The listing builds one solid part. Answer for the finished solid, in the listing's coordinates (mm). Give positions to 0.01 mm unless a question says otherwise; leave off trailing zeros. Write each loop counter-clockwise with the first axis right and the second up, starting at its lowest first coordinate (ties: lowest second). Pieces come first, ordered by that corner, then holes.
```python
from build123d import *

# Parameters (mm, degrees)
SKETCH1_R           = 1.5
BOSS_EXTRUDE1_DEPTH = 2
FILLET1_R           = 8


with BuildPart() as part:
    # Sketch1 → Boss-Extrude1 (new body)
    with BuildSketch(Plane.XY):
        with BuildLine():
            Line((85, 40), (85, -45))
            Line((85, -45), (58.094750193, -45))
            ThreePointArc((58.094750193, -45), (0, -30), (-58.094750193, -45))
            Line((-58.094750193, -45), (-85, -45))
            Line((-85, -45), (-85, 40))
            ThreePointArc((-85, 40), (-74.748737342, 64.748737342), (-50, 75))
            Line((-50, 75), (50, 75))
            ThreePointArc((50, 75), (74.748737342, 64.748737342), (85, 40))
        make_face()
        with Locations((50, 55)):
            Circle(SKETCH1_R, mode=Mode.SUBTRACT)
        with Locations((-75, -38)):
            Circle(SKETCH1_R, mode=Mode.SUBTRACT)
        with Locations((75, -38)):
            Circle(SKETCH1_R, mode=Mode.SUBTRACT)
        with Locations((-50, 55)):
            Circle(SKETCH1_R, mode=Mode.SUBTRACT)
        with BuildLine():
            ThreePointArc((-22.15, 67.8), (-20, 65.65), (-17.85, 67.8))
            Line((-17.85, 67.8), (-17.85, 71))
            ThreePointArc((-17.85, 71), (-20, 73.15), (-22.15, 71))
            Line((-22.15, 71), (-22.15, 67.8))
        make_face(mode=Mode.SUBTRACT)
        with BuildLine():
            Line((81, 15.701693023), (77.8, 15.701693023))
            ThreePointArc((77.8, 15.701693023), (75.651693023, 17.85), (77.8, 19.998306977))
            Line((77.8, 19.998306977), (81, 19.998306977))
            ThreePointArc((81, 19.998306977), (83.148306977, 17.85), (81, 15.701693023))
        make_face(mode=Mode.SUBTRACT)
        with BuildLine():
            Line((-81, -15.701693023), (-77.8, -15.701693023))
            ThreePointArc((-77.8, -15.701693023), (-75.651693023, -17.85), (-77.8, -19.998306977))
            Line((-77.8, -19.998306977), (-81, -19.998306977))
            ThreePointArc((-81, -19.998306977), (-83.148306977, -17.85), (-81, -15.701693023))
        make_face(mode=Mode.SUBTRACT)
        with BuildLine():
            ThreePointArc((-77.8, 15.701693023), (-75.651693023, 17.85), (-77.8, 19.998306977))
            Line((-77.8, 19.998306977), (-81, 19.998306977))
            ThreePointArc((-81, 19.998306977), (-83.148306977, 17.85), (-81, 15.701693023))
            Line((-81, 15.701693023), (-77.8, 15.701693023))
        make_face(mode=Mode.SUBTRACT)
        with BuildLine():
            ThreePointArc((77.8, -15.701693023), (75.651693023, -17.85), (77.8, -19.998306977))
            Line((77.8, -19.998306977), (81, -19.998306977))
            ThreePointArc((81, -19.998306977), (83.148306977, -17.85), (81, -15.701693023))
            Line((81, -15.701693023), (77.8, -15.701693023))
        make_face(mode=Mode.SUBTRACT)
        with BuildLine():
            Line((22.15, 71), (22.15, 67.8))
            ThreePointArc((22.15, 67.8), (20, 65.65), (17.85, 67.8))
            Line((17.85, 67.8), (17.85, 71))
            ThreePointArc((17.85, 71), (20, 73.15), (22.15, 71))
        make_face(mode=Mode.SUBTRACT)
    extrude(amount=BOSS_EXTRUDE1_DEPTH)

    # Fillet1
    fillet1_edges = [part.edges().sort_by_distance(p)[0] for p in [
        (85, -45, 1),
        (-85, -45, 1),
    ]]
    fillet(fillet1_edges, radius=FILLET1_R)


solid = part.part
```
Item 1: A cutting plane is placed at A-A, the plane y = -17.85. Give the vertices of the cut face in (x, z), plus the area to 3 significant figures.
Conclusion:
outline: (-85, 0) - (-83.15, 0) - (-83.15, 2) - (-85, 2) - close; (-75.65, 0) - (75.65, 0) - (75.65, 2) - (-75.65, 2) - close; (83.15, 0) - (85, 0) - (85, 2) - (83.15, 2) - close
area: 310 mm2
Item 2: A cutting plane is placed at B-B, the plane z = 1.25. Count the separate pieces of the cut face and the enclosed holes in it, plus the area to 3 significant figures.
Conclusion:
separate pieces: 1
enclosed holes: 10
area: 18,500 mm2
Item 3: A cutting plane is placed at D-D, the plane y = 50.5. Give the vertices of the cut face in (x, z).
Conclusion:
outline: (-83.39, 0) - (83.39, 0) - (83.39, 2) - (-83.39, 2) - close
Item 4: Each of these flat-tipped pins is pushed along its axis until it touches: P1, Ø1, axis at x = 80, z = 1, coming from the -Y side; P2, Ø1, axis at y = 70, z = 1.5, coming from the +X side; P3, Ø0.6, axis at x = -79.5, z = 1, coming from the -Y side. Where does it stop, or does it pass through?
Conclusion:
P1: stops at y = -44.6
P2: stops at x = 68.83
P3: stops at y = -44.69
Item 5: Determine the mould class of faces 1 (the face through (74.475, 65.019, 0.986)), 2 (the face through (0.849, -30.003, 0.986)), 3 (the face through (-75.019, 64.475, 0.986)), 4 (the face through (1, 16, 0)) for opening direction X: pulls with the +X half, pulls with the -X half, needs draft (parallel to the pull), parting line crosses it, or undercut.
Conclusion:
face 1: pulls with the +X half
face 2: undercut
face 3: pulls with the -X half
face 4: needs draft
Item 6: A cutting plane is placed at C-C, the plane x = 7. Give the vertices of the cut face in (y, z), plus the area to 3 significant figures.
Conclusion:
outline: (-30.2, 0) - (75, 0) - (75, 2) - (-30.2, 2) - close
area: 210 mm2
Item 7: Consider probe 1 along Y at (x, z) = (77, 1.9); probe 2 along Y at (x, z) = (75, 1.3); probe 3 along Y at (x, z) = (20, 0.75). Determine where each line is inside the solid, lowest interval first.
Conclusion:
probe 1: y = -45 to -19.84, -15.86 to 15.86, 19.84 to 62.27
probe 2: y = -45 to -39.5, -36.5 to 64.49
probe 3: y = -31.68 to 65.65, 73.15 to 75
